```python
from build123d import *

# Parameters (mm, degrees)
F0_R     = 17.2972377105
F1_DEPTH = 76.2
F2_SIZE2 = 26.1697224203
F2_SIZE  = 9.525
F3_R     = 6.35
F4_R     = 19.4529047129
F5_DEPTH = 1.27


with BuildPart() as f1:
    # F0 (on Front) → F1 (new body)
    with BuildSketch(Plane.XZ):
        Circle(F0_R)
    extrude(amount=F1_DEPTH)

    # F2
    f2_edges = [f1.edges().sort_by_distance(p)[0] for p in [
        (-17.297238, -76.2, 0),
    ]]
    f2_side = f1.faces().sort_by_distance((0, -76.2, 0))[0]
    chamfer(f2_edges, length=F2_SIZE, length2=F2_SIZE2, reference=f2_side)

    # F3
    f3_edges = [f1.edges().sort_by_distance(p)[0] for p in [
        (-7.772238, -76.2, 0),
    ]]
    fillet(f3_edges, radius=F3_R)

    # F4 (on face) → F5 (join)
    with BuildSketch(Plane(origin=(0, 0, 0), x_dir=(-1, 0, 0), z_dir=(0, 1, 0))):
        Circle(F4_R)
    extrude(amount=F5_DEPTH)


solid = f1.part
```
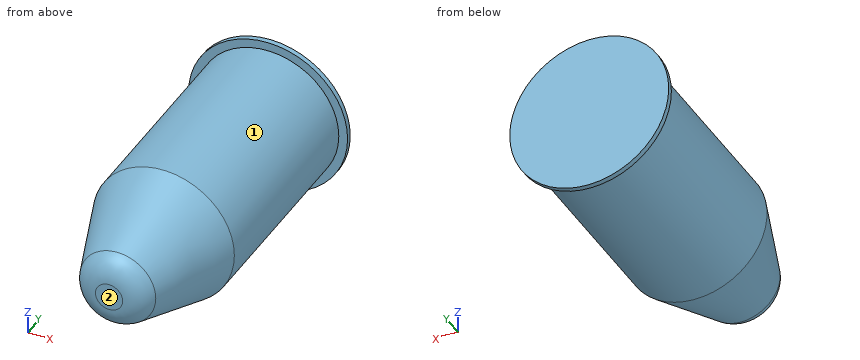
Input: part model. Units: mm. Frame: model coordinates. Face numbers are marked on the shaded views. A direction names the side the tool comes from. Give positions to 0.01 mm unless a question says otherwise; leave off trailing zeros. Loops run counter-clockwise (first coordinate to the right, second up) from the corner with the lowest first, then second, coordinate; pieces in that order, holes last. Notation, with made-up numbers: M 14,-21 L 47,-21 A15 cw 47,3 Z; hole C 25,0 d4. An arc over 180 degrees is marked long. Answer as CSV lines item,"result". Start each with the question number.
1. Section B-B on y = -56.5. Return loops of the section in (x, z).
2. Line query: L1, parallel to Y at x = 14.5, z = -12; L2, parallel to X at y = -11, z = -0.5; L3, parallel to Z at x = -11, y = -47. Output: solid intervals per line, ascending.
3. Pin query (flat end, axial travel): P1, Ø4, axis at y = -61.5, z = 13.5, coming from the -X side; P2, Ø1, axis at x = -9, y = -42, coming from the +Z side; P3, Ø2, axis at x = -1.5, y = -14, coming from the -Z side; P4, Ø11.5, axis at x = 0.5, z = -6.5, coming from the -Y side. Return the tip coordinate at first contact, or that it passes through.
4. Section A-A on y = -9. Return loops of the section in (x, z).
5. Reachability of the marked faces 1 and 2 from +Z, -Z, +X, -X, +Y, -Y: full face, straight path, thin tool, end or side. Return the list, or none.
Computed values:
1,outline,"C 0,0 d29.88"
2,L1,"y = 0 to 1.27"
2,L2,"x = -17.29 to 17.29"
2,L3,"z = -13.35 to 13.35"
3,P1,"stops at x = -6.62"
3,P2,"stops at z = 15.06"
3,P3,"stops at z = -17.29"
3,P4,"stops at y = -76.2"
4,outline,"C 0,0 d34.59"
5,face 1,"-Y"
5,face 2,"+Z, -Z, +X, -X, -Y"
